```python
from build123d import *

# Parameters (mm, degrees)
SKETCH1_W           = 26
SKETCH1_H           = 100
BOSS_EXTRUDE1_DEPTH = 6.35
SKETCH2_W           = 22
SKETCH2_H           = 42.6
CUT_EXTRUDE1_DEPTH  = 84.596948906
HOLE1_D             = 4.25


with BuildPart() as part:
    # Sketch1 → Boss-Extrude1 (new body)
    with BuildSketch(Plane(origin=(0, 0, 7.302957559), x_dir=(-1, 0, 0), z_dir=(0, 0, -1))):
        with Locations((14.325270249, 28.74932998)):
            Rectangle(SKETCH1_W, SKETCH1_H)
    extrude(amount=BOSS_EXTRUDE1_DEPTH)

    # Sketch2 → Cut-Extrude1 (cut, through all)
    with BuildSketch(Plane(origin=(0, 0, 0.952957559), x_dir=(-1, 0, 0), z_dir=(0, 0, -1))):
        with Locations((14.325270249, 49.44932998)):
            Rectangle(SKETCH2_W, SKETCH2_H)
    extrude(amount=-CUT_EXTRUDE1_DEPTH, mode=Mode.SUBTRACT)

    # Hole1 (through all)
    with Locations(Plane.XY.offset(7.302957559)):
        with Locations((-19.225270249, 73.24932998), (-9.225270249, 73.24932998), (-19.225270249, 24.94932998), (-9.225270249, 24.94932998)):
            Hole(HOLE1_D / 2)


solid = part.part
```
The model under review builds one solid part; all positions refer to its coordinate system, in mm. A direction names the side the tool comes from. Round coordinates to 2 decimals unless told otherwise and drop trailing zeros. Loops run counter-clockwise (first coordinate to the right, second up) from the corner with the lowest first, then second, coordinate; pieces in that order, holes last. Notation, with made-up numbers: (-11.5, -20) -> (43.5, -20) arc R15 cw to (43.5, -5) -> close; hole circle Ø5 at (-16.75, -22). An arc over 180 degrees is marked (long way). Answer as a JSON object with one key per item and string values. Group by question number.
1) For faces 4 (the face through (-3.325, 49, 4)), 5 (the face through (-14, 18, 7.303)), list the 3-axis set-ups (+Z, -Z, +X, -X, +Y, -Y) from which the entire face can be reached by the end or side of a thin tool; tool diameter is ignored.
2) For line 1 (Y direction, x = -9, z = 5.75); line 2 (X direction, y = 60.5, z = 3); line 3 (Y direction, x = -10.25, z = 1.75), list the stretches that pass through material, from the lowest coordinate up. Write a range as [from, to].
3) For pin 1 Ø3.5 at (x, y) = (-9.23, 24.95) entering from -Z, flat-tipped, find the tip position at first contact; note if it passes through.
4) Mouldability with a two-part tool opening along Y and no side actions: class faces 1 (the face through (-8.765, 71.175, 4.084)), 2 (the face through (-14, -21.251, 4)), 3 (the face through (-1.325, 28, 4)) as released by +Y, released by -Y, zero draft, split by the parting line, or undercut.
5) We need section C-C on z = 5. Write out the cut boundary in (x, y) (3 decimals).
6) We need section D-D on x = -8.75. Write out the cut boundary in (y, z).
7) We need section A-A on y = 65. Write out the cut boundary in (x, z).
8) We need section B-B on x = -18.5. Write out the cut boundary in (y, z), then the cut area to 3 significant figures.
Result set:
{
 "1": {"face 4": "+Z, -Z", "face 5": "+Z, +X, -X, +Y, -Y"},
 "2": {"line 1": "[-21.25, 22.84], [27.06, 28.15], [70.75, 71.14], [75.36, 78.75]", "line 2": "[-27.33, -25.33], [-3.33, -1.33]", "line 3": "[-21.25, 23.09], [26.81, 28.15], [70.75, 71.39], [75.11, 78.75]"},
 "3": {"pin 1": "through"},
 "4": {"face 1": "undercut", "face 2": "released by -Y", "face 3": "zero draft"},
 "5": {"outline": "(-27.325, -21.251) -> (-1.325, -21.251) -> (-1.325, 78.749) -> (-27.325, 78.749) -> close; hole (-25.325, 28.149) -> (-3.325, 28.149) -> (-3.325, 70.749) -> (-25.325, 70.749) -> close; hole circle Ø4.25 at (-19.225, 24.949); hole circle Ø4.25 at (-19.225, 73.249); hole circle Ø4.25 at (-9.225, 24.949); hole circle Ø4.25 at (-9.225, 73.249)"},
 "6": {"outline": "(-21.25, 0.95) -> (22.88, 0.95) -> (22.88, 7.3) -> (-21.25, 7.3) -> close; (27.02, 0.95) -> (28.15, 0.95) -> (28.15, 7.3) -> (27.02, 7.3) -> close; (70.75, 0.95) -> (71.18, 0.95) -> (71.18, 7.3) -> (70.75, 7.3) -> close; (75.32, 0.95) -> (78.75, 0.95) -> (78.75, 7.3) -> (75.32, 7.3) -> close"},
 "7": {"outline": "(-27.33, 0.95) -> (-25.33, 0.95) -> (-25.33, 7.3) -> (-27.33, 7.3) -> close; (-3.33, 0.95) -> (-1.33, 0.95) -> (-1.33, 7.3) -> (-3.33, 7.3) -> close"},
 "8": {"outline": "(-21.25, 0.95) -> (22.95, 0.95) -> (22.95, 7.3) -> (-21.25, 7.3) -> close; (26.95, 0.95) -> (28.15, 0.95) -> (28.15, 7.3) -> (26.95, 7.3) -> close; (70.75, 0.95) -> (71.25, 0.95) -> (71.25, 7.3) -> (70.75, 7.3) -> close; (75.25, 0.95) -> (78.75, 0.95) -> (78.75, 7.3) -> (75.25, 7.3) -> close", "area": "314 mm²"}
}
